from build123d import *

# Parameters (mm, degrees)
EXTRUDE_1_DEPTH     = 3
CUT_EXTRUDE_1_REACH = 5
SKETCH_2_R          = 6.1
SKETCH_2_W          = 36
SKETCH_2_H          = 36
MM_CLEARANCE_1_D    = 3
MM_CLEARANCE_4_D    = 3
MM_PRESS_1_D        = 3
MM_PRESS_2_D        = 3
MM_PRESS_4_D        = 3


with BuildPart() as part:
    # 草图1 → 凸台-拉伸1 (new body)
    with BuildSketch(Plane.XY):
        with BuildLine():
            Line((30.58739299, 31.55542954), (153.948275504, 31.55542954))
            Line((153.948275504, 31.55542954), (184.822670137, -29.838251263))
            ThreePointArc((184.822670137, -29.838251263), (183.892664178, -36.470729041), (178.540104648, -40.496245038))
            ThreePointArc((178.540104648, -40.496245038), (162.746691749, -43.998966844), (146.755444956, -46.44457046))
            Line((146.755444956, -46.44457046), (49.675444956, -46.44457046))
            Line((49.675444956, -46.44457046), (49.675444956, -2.44457046))
            Line((49.675444956, -2.44457046), (23.694682842, 12.55542954))
            Line((23.694682842, 12.55542954), (3.843759809, 14.992816408))
            Line((3.843759809, 14.992816408), (5.87739299, 31.55542954))
            Line((5.87739299, 31.55542954), (30.58739299, 31.55542954))
        make_face()
    extrude(amount=EXTRUDE_1_DEPTH)

    # 草图2 → 切除-拉伸1 (cut, up to next)
    with BuildSketch(Plane.XY.offset(3), mode=Mode.PRIVATE) as cut_extrude_1_sk1:
        with Locations((173.675444956, -31.44457046)):
            Circle(SKETCH_2_R)
    cut_extrude_1_tool1 = extrude(cut_extrude_1_sk1.sketch, amount=-CUT_EXTRUDE_1_REACH, mode=Mode.PRIVATE) & part.part
    add(cut_extrude_1_tool1.solids().sort_by_distance((173.675445, -31.44457, 3))[0], mode=Mode.SUBTRACT)
    # 草图2 → 切除-拉伸1 (cut, up to next)
    with BuildSketch(Plane.XY.offset(3), mode=Mode.PRIVATE) as cut_extrude_1_sk2:
        with Locations((83.439887491, -4.827295438)):
            Rectangle(SKETCH_2_W, SKETCH_2_H)
    cut_extrude_1_tool2 = extrude(cut_extrude_1_sk2.sketch, amount=-CUT_EXTRUDE_1_REACH, mode=Mode.PRIVATE) & part.part
    add(cut_extrude_1_tool2.solids().sort_by_distance((83.439887, -4.827295, 3))[0], mode=Mode.SUBTRACT)
    # 草图2 → 切除-拉伸1 (cut, up to next)
    with BuildSketch(Plane.XY.offset(3), mode=Mode.PRIVATE) as cut_extrude_1_sk3:
        Polygon((112.439887491, -4.827295438), (112.439887491, -33.327295438), (120.439887491, -33.327295438), (120.439887491, 23.672704562), (112.439887491, 23.672704562), align=None)
    cut_extrude_1_tool3 = extrude(cut_extrude_1_sk3.sketch, amount=-CUT_EXTRUDE_1_REACH, mode=Mode.PRIVATE) & part.part
    add(cut_extrude_1_tool3.solids().sort_by_distance((116.439887, -4.827295, 3))[0], mode=Mode.SUBTRACT)

    # 大小mm Clearance 暗销孔1 (through all)
    with Locations(Plane(origin=(141.510624827, 151.85923203, 3), x_dir=(-0.999780146, -0.020968043, 0), z_dir=(0, 0, 1))):
        with Locations((20.591231353, 123.39816829), (42.591231353, 122.936763059), (64.581557509, 122.475560716)):
            Hole(MM_CLEARANCE_1_D / 2)

    # 大小mm Clearance 暗销孔4 (through all)
    with Locations(Plane(origin=(141.510624827, 151.85923203, 3), x_dir=(-0.999780146, -0.020968043, 0), z_dir=(0, 0, 1))):
        with Locations((20.608818994, 135.452556109), (-0.900285243, 135.452556109)):
            Hole(MM_CLEARANCE_4_D / 2)

    # 大小mm Press 暗销孔1 (through all)
    with Locations(Plane(origin=(141.673702765, 151.858231724, 3), x_dir=(-0.99978014, -0.020968354, 0), z_dir=(0, 0, 1))):
        with Locations((36.045400202, 133.709111751), (36.930668673, 175.919093371)):
            Hole(MM_PRESS_1_D / 2)

    # 大小mm Press 暗销孔2 (through all)
    with Locations(Plane(origin=(143.54728393, 150.625368255, 3), x_dir=(-0.99975237, -0.022253058, 0), z_dir=(0, 0, 1))):
        with Locations((88.938953066, 135.227377046), (101.942467158, 126.647536361), (127.53759353, 125.598807912), (135.454300746, 124.4473971)):
            Hole(MM_PRESS_2_D / 2)

    # 大小mm Press 暗销孔4 (through all)
    with Locations(Plane(origin=(143.54728393, 150.625368255, 3), x_dir=(-0.99975237, -0.022253058, 0), z_dir=(0, 0, 1))):
        with Locations((93.161367469, 190.578219389), (93.161367469, 182.547127137), (40.245392963, 190.578219389), (40.245392963, 182.547127137)):
            Hole(MM_PRESS_4_D / 2)


solid = part.part
Model file for the job. Use its own axes, mm. A direction names the side the tool comes from. Give positions to 0.01 mm unless a question says otherwise; leave off trailing zeros. Order: outer loops, then holes, each group sorted by start corner. A loop starts at its lowest first (then second) coordinate and runs counter-clockwise, first axis right, second up. Notation, with made-up numbers: (61, 17) - (73, 17) arc R28 ccw to (73, 53) - close; hole circle Ø3 at (-26, 25). An arc over 180 degrees is marked (long way). One line per item, written item: value.
Item 1: Tool access for faces 1 (the flat face through (49.675, -25, 1)), 2 (the flat face through (79, 31.555, 1)), 3 (the flat face through (120.44, -5, 2)): list every direction of +Z, -Z, +X, -X, +Y, -Y with a clear straight run to the whole face (end or side of a thin tool).
Response values:
face 1: +Z, -Z, -X, -Y
face 2: +Z, -Z, +X, -X, +Y
face 3: +Z, -Z
Item 2: Slice it at C-C (z = 1.65). Give the number of separate pieces and of enclosed holes in the cut face, then the cut area to 3 significant figures.
Response values:
separate pieces: 1
enclosed holes: 18
area: 8,510 mm2
Item 3: Slice it at D-D (y = -21). List the corners of the cut face in (x, z).
Response values:
outline: (49.68, 0) - (65.44, 0) - (65.44, 3) - (49.68, 3) - close; (101.44, 0) - (112.44, 0) - (112.44, 3) - (101.44, 3) - close; (120.44, 0) - (180.38, 0) - (180.38, 3) - (120.44, 3) - close
Item 4: Wall check: line 1 (Y direction, x = 97.5, z = 2.75); line 2 (X direction, y = 0, z = 1.3); line 3 (X direction, y = -34.5, z = 0.4). Give the ranges that are in metal, low to high.
Response values:
line 1: -46.44 to -22.83, 13.17 to 31.56
line 2: 45.44 to 65.44, 101.44 to 112.44, 120.44 to 169.82
line 3: 49.68 to 53.08, 55.87 to 168.4, 178.96 to 184.75
Item 5: Slice it at B-B (y = -7.5). List the corners of the cut face in (x, z), then the cut area to 3 significant figures.
Response values:
outline: (49.68, 0) - (65.44, 0) - (65.44, 3) - (49.68, 3) - close; (101.44, 0) - (112.44, 0) - (112.44, 3) - (101.44, 3) - close; (120.44, 0) - (173.59, 0) - (173.59, 3) - (120.44, 3) - close
area: 240 mm2
Item 6: Two-plate mould, pull along Y, no slides. Class faces 4 (the flat face through (99, -46.445, 1)), 5 (the flat face through (169.17, 1.29, 1.48)), 6 (the flat face through (65.44, -5, 2)), 7 (the cylindrical face through (108.22, -39.46, 1.48)): released by +Y, released by -Y, zero draft, split by the parting line, or undercut.
Response values:
face 4: released by -Y
face 5: released by +Y
face 6: undercut
face 7: undercut
Item 7: Pin check, flat tips, straight feed: pin 1 Ø2.5 at (x, y) = (101.51, 28.06) entering from -Z; pin 2 Ø5 at (x, y) = (54.65, -41.98) entering from -Z; pin 3 Ø1.5 at (y, z) = (-7, 1.5) entering from +X; pin 4 Ø1.5 at (y, z) = (-24, 2.5) entering from +X. Stop position of each tip, or through.
Response values:
pin 1: through
pin 2: z = 0
pin 3: x = 173.71
pin 4: x = 182.26
Item 8: Slice it at A-A (x = 86.5). List the corners of the cut face in (y, z), then the cut area to 3 significant figures.
Response values:
outline: (-46.44, 0) - (-22.83, 0) - (-22.83, 3) - (-46.44, 3) - close; (13.17, 0) - (31.56, 0) - (31.56, 3) - (13.17, 3) - close
area: 126 mm2
